```python
from build123d import *

# Parameters (mm, degrees)
ENL_V_MAT_EXTRU_1_DEPTH = 12.5


with BuildPart() as part:
    # Esquisse1 → Révolution1 (revolve)
    with BuildSketch(Plane(origin=(0, 0, 0), x_dir=(0, 0, -1), z_dir=(1, 0, 0)), mode=Mode.PRIVATE) as r_volution1_sk:
        Polygon((73.269946074, 13.728692904), (72.036236822, 13.728692904), (58.269946074, 11.228692904), (23.269946074, 11.228692904), (23.269946074, 7.228692904), (63.269946074, 7.228692904), (63.269946074, 10.228692904), (73.269946074, 10.228692904), align=None)
    revolve(r_volution1_sk.sketch.rotate(Axis((0, 7.228692904, -23.269946074), (0, 0, -1)), 90), axis=Axis((0, 7.228692904, -23.269946074), (0, 0, -1)))

    # Esquisse12 → Enlèv. mat.-Extru.1 (cut)
    with BuildSketch(Plane(origin=(0, 0, -73.269946074), x_dir=(-1, 0, 0), z_dir=(0, 0, -1))):
        Polygon((0.5, 7.728692904), (6.052650367, 7.728692904), (6.052650367, 6.728692904), (0.5, 6.728692904), (0.5, 2.030323732), (-0.5, 2.030323732), (-0.5, 6.728692904), (-5.684461256, 6.728692904), (-5.684461256, 7.728692904), (-0.5, 7.728692904), (-0.5, 12.693209271), (0.5, 12.693209271), align=None)
    extrude(amount=-ENL_V_MAT_EXTRU_1_DEPTH, mode=Mode.SUBTRACT)


solid = part.part
```
Source: CAD feature listing. Evaluate the final solid. Frame: model axes, mm. A direction names the side the tool comes from. Give positions to 0.01 mm unless a question says otherwise; leave off trailing zeros. Loops run counter-clockwise (first coordinate to the right, second up) from the corner with the lowest first, then second, coordinate; pieces in that order, holes last. Notation, with made-up numbers: (38.25, -27) -> (91.25, -27) arc R37 cw to (91.25, 9) -> close; hole circle Ø8 at (33, 66). An arc over 180 degrees is marked (long way). Use a Markdown table: item, result. Add a question column.
(1) Section query A-A (x = 0). Output: boundary loops of the cut face in (y, z).
(2) Pull-direction query (Y, two-part tool) for faces 1 (the face through (0, 7, -23.27)), 2 (the face through (-0.5, 4, -66)), 3 (the face through (4.726, 5.74, -63.527)); classes: +Y half, -Y half, draft (parallel to the pull), parting line (faces both ways), or undercut.
(3) Ray query, line 1 (X direction, y = 7.5, z = -52); line 2 (Z direction, x = 1, y = 6); line 3 (X direction, y = 6.5, z = -67). Return the intervals inside material, ascending.
(4) Access query for faces 4 (the face through (-2.103, 5.089, -68.34)), 5 (the face through (5.684, 7, -70)). Directions: +Z, -Z, +X, -X, +Y, -Y. A direction counts if a zero-diameter tool reaches every point of the face in a straight line with its end or side. Return the directions, or none.
(5) First-contact query: pin 1 Ø1.7 at (x, z) = (-2, -68.5) entering from +Y; pin 2 Ø4.5 at (x, z) = (-4, -70) entering from -Y; pin 3 Ø6 at (x, z) = (3.5, -43) entering from +Y; pin 4 Ø3 at (x, y) = (5, 12) entering from -Z. Flat tips, straight axial feed; report the tip coordinate or a pass-through.
(6) Section query C-C (z = -46). Output: boundary loops of the cut face in (x, y), then the cut area to 3 significant figures.
(7) Section query B-B (z = -62). Output: boundary loops of the cut face in (x, y), then the cut area to 3 significant figures.
Checked values:
| question | item | result |
|---|---|---|
| 1 | outline | (0.73, -73.27) -> (2.03, -73.27) -> (2.03, -64.87) -> (0.73, -72.04) -> close; (2.77, -60.77) -> (11.68, -60.77) -> (11.23, -58.27) -> (11.23, -23.27) -> (3.23, -23.27) -> (3.23, -58.27) -> close; (12.69, -73.27) -> (13.73, -73.27) -> (13.73, -72.04) -> (12.69, -66.33) -> close |
| 2 | face 1 | draft |
| 2 | face 2 | undercut |
| 2 | face 3 | parting line |
| 3 | line 1 | -3.99 to 3.99 |
| 3 | line 2 | -63.27 to -23.27 |
| 3 | line 3 | -5.54 to -2.91, 2.91 to 5.54 |
| 4 | face 4 | -Z |
| 4 | face 5 | +Z, -Z |
| 5 | pin 1 | y = 13.03 |
| 5 | pin 2 | y = 1.24 |
| 5 | pin 3 | y = 11.2 |
| 5 | pin 4 | z = -73.27 |
| 6 | outline | circle Ø8 at (0, 7.23) |
| 6 | area | 50.3 mm^2 |
| 7 | outline | (-4.65, 6.73) arc R4.68 ccw to (-0.5, 2.58) -> (-0.5, 6.73) -> close; (-4.65, 7.73) -> (-0.5, 7.73) -> (-0.5, 11.88) arc R4.68 ccw to start; (0.5, 2.58) arc R4.68 ccw to (4.65, 6.73) -> (0.5, 6.73) -> close; (0.5, 7.73) -> (4.65, 7.73) arc R4.68 ccw to (0.5, 11.88) -> close |
| 7 | area | 51.1 mm^2 |
